```python
from build123d import *

# Parameters (mm, degrees)
EXTRUDE_1_DEPTH     = 47
SKETCH_2_R          = 11
EXTRUDE_2_DEPTH     = 2
SKETCH_3_R          = 4
EXTRUDE_3_DEPTH     = 45
SKETCH_6_R          = 1.5
CUT_EXTRUDE_2_DEPTH = 3.5


with BuildPart() as part:
    # 草图1 → 凸台-拉伸1 (new body)
    with BuildSketch(Plane.XY):
        with BuildLine():
            Line((18, -21), (-18, -21))
            ThreePointArc((-18, -21), (-20.121320344, -20.121320344), (-21, -18))
            Line((-21, -18), (-21, 18))
            ThreePointArc((-21, 18), (-20.121320344, 20.121320344), (-18, 21))
            Line((-18, 21), (18, 21))
            ThreePointArc((18, 21), (20.121320344, 20.121320344), (21, 18))
            Line((21, 18), (21, -18))
            ThreePointArc((21, -18), (20.121320344, -20.121320344), (18, -21))
        make_face()
    extrude(amount=EXTRUDE_1_DEPTH)

    # 草图2 → 凸台-拉伸2 (add)
    with BuildSketch(Plane.XY.offset(47)):
        Circle(SKETCH_2_R)
    extrude(amount=EXTRUDE_2_DEPTH)

    # 草图3 → 凸台-拉伸3 (add)
    with BuildSketch(Plane.XY.offset(49)):
        with Locations(Location((0, 0, 0), (0, 0, 180))):
            Circle(SKETCH_3_R)
    extrude(amount=EXTRUDE_3_DEPTH)

    # 草图6 → 切除-拉伸2 (cut)
    with BuildSketch(Plane.XY.offset(47)):
        with Locations((-15.5, 15.5)):
            Circle(SKETCH_6_R)
        with Locations((15.5, 15.5)):
            Circle(SKETCH_6_R)
        with Locations((15.5, -15.5)):
            Circle(SKETCH_6_R)
        with Locations((-15.5, -15.5)):
            Circle(SKETCH_6_R)
    extrude(amount=-CUT_EXTRUDE_2_DEPTH, mode=Mode.SUBTRACT)


solid = part.part
```
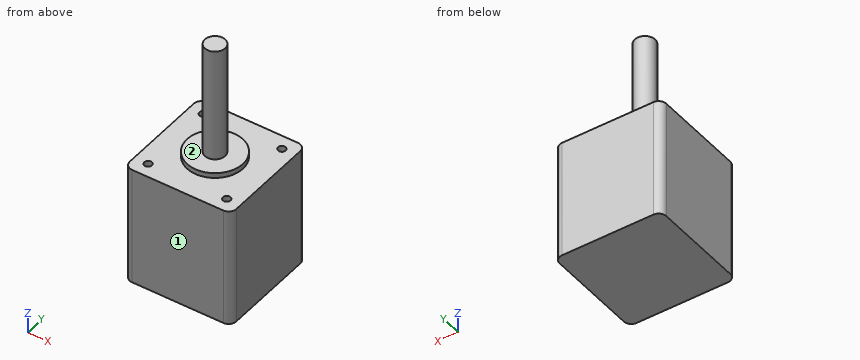
Check sheet for the modelled part. Datum: model origin and axes. Units: mm. Face numbers are marked on the shaded views. A direction names the side the tool comes from. Round coordinates to 2 decimals unless told otherwise and drop trailing zeros. Write each loop counter-clockwise with the first axis right and the second up, starting at its lowest first coordinate (ties: lowest second). Pieces come first, ordered by that corner, then holes. Notation, with made-up numbers: (85.25, 7) -> (138.25, 7) arc R23 cw to (138.25, 33) -> close; hole circle Ø9 at (48.5, 63.5). An arc over 180 degrees is marked (long way). Put each result on its own line as item: value.
(1) Go/stop test with flat-tipped pins: pin 1 Ø0.9 at (x, y) = (15, 15) entering from +Z; pin 2 Ø2 at (x, z) = (3, 50.5) entering from -Y; pin 3 Ø3.5 at (x, y) = (15, -15.5) entering from +Z. Record where each tip stops, or that it passes through.
Values found:
pin 1: stops at z = 43.5
pin 2: stops at y = -3.46
pin 3: stops at z = 47
(2) Material ranges on line 1 (Y direction, x = 15.5, z = 45); line 2 (Y direction, x = 15, z = 46), recorded low to high.
Values found:
line 1: y = -21 to -17, -14 to 14, 17 to 21
line 2: y = -21 to -16.91, -14.09 to 14.09, 16.91 to 21
(3) Sectioned sample at D-D (y = 6). Enter the section's corners in (x, z).
Values found:
outline: (-21, 0) -> (21, 0) -> (21, 47) -> (9.22, 47) -> (9.22, 49) -> (-9.22, 49) -> (-9.22, 47) -> (-21, 47) -> close
(4) Sectioned sample at C-C (z = 79). Enter the section's corners in (x, y).
Values found:
outline: circle Ø8 at (0, 0)
(5) Tool access check on the marked faces 1 and 2. Record the directions out of +Z, -Z, +X, -X, +Y, -Y that give a thin tool (end or side, any length) a straight path to the whole face; none if there is none.
Values found:
face 1: +Z, -Z, +X, -X, -Y
face 2: +Z
(6) Sectioned sample at A-A (y = 15.5). Enter the section's corners in (x, z).
Values found:
outline: (-21, 0) -> (21, 0) -> (21, 47) -> (17, 47) -> (17, 43.5) -> (14, 43.5) -> (14, 47) -> (-14, 47) -> (-14, 43.5) -> (-17, 43.5) -> (-17, 47) -> (-21, 47) -> close
